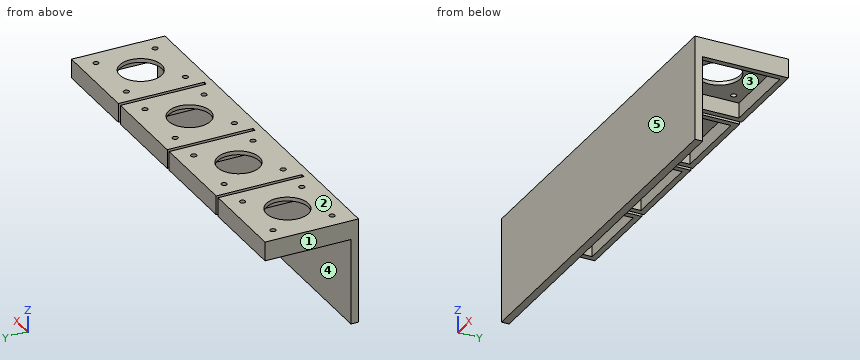
```python
from build123d import *

# Parameters (mm, degrees)
SKETCH_1_W           = 48
SKETCH_1_H           = 48
SKETCH_1_W_2         = 42
SKETCH_1_H_2         = 42
EXTRUDE_1_DEPTH      = 10
EXTRUDE_1_2_DEPTH    = 10
EXTRUDE_1_3_DEPTH    = 10
EXTRUDE_1_4_DEPTH    = 10
SKETCH_2_W           = 42
SKETCH_2_H           = 42
SKETCH_2_R           = 1.45
SKETCH_2_R_2         = 11
EXTRUDE_2_DEPTH      = 2
SKETCH_3_W           = 198
SKETCH_3_H           = 55
EXTRUDE_3_DEPTH      = 1
EXTRUDE_3_DEPTH_BACK = 3


with BuildPart() as part:
    # Sketch 1 → Extrude 1 (new body)
    with BuildSketch(Plane.XY):
        Rectangle(SKETCH_1_W, SKETCH_1_H)
        Rectangle(SKETCH_1_W_2, SKETCH_1_H_2, mode=Mode.SUBTRACT)
    extrude(amount=EXTRUDE_1_DEPTH)

    # Sketch 2 → Extrude 2 (add)
    with BuildSketch(Plane.XY.offset(10)):
        Rectangle(SKETCH_2_W, SKETCH_2_H)
        with Locations((-15.5, 15.5)):
            Circle(SKETCH_2_R, mode=Mode.SUBTRACT)
        with Locations((15.5, 15.5)):
            Circle(SKETCH_2_R, mode=Mode.SUBTRACT)
        with Locations((15.5, -15.5)):
            Circle(SKETCH_2_R, mode=Mode.SUBTRACT)
        with Locations((-15.5, -15.5)):
            Circle(SKETCH_2_R, mode=Mode.SUBTRACT)
        Circle(SKETCH_2_R_2, mode=Mode.SUBTRACT)
        with Locations((50, 0)):
            Rectangle(SKETCH_2_W, SKETCH_2_H)
        with Locations((34.5, 15.5)):
            Circle(SKETCH_2_R, mode=Mode.SUBTRACT)
        with Locations((65.5, 15.5)):
            Circle(SKETCH_2_R, mode=Mode.SUBTRACT)
        with Locations((65.5, -15.5)):
            Circle(SKETCH_2_R, mode=Mode.SUBTRACT)
        with Locations((34.5, -15.5)):
            Circle(SKETCH_2_R, mode=Mode.SUBTRACT)
        with Locations((50, 0)):
            Circle(SKETCH_2_R_2, mode=Mode.SUBTRACT)
        with Locations((100, 0)):
            Rectangle(SKETCH_2_W, SKETCH_2_H)
        with Locations((84.5, 15.5)):
            Circle(SKETCH_2_R, mode=Mode.SUBTRACT)
        with Locations((115.5, 15.5)):
            Circle(SKETCH_2_R, mode=Mode.SUBTRACT)
        with Locations((115.5, -15.5)):
            Circle(SKETCH_2_R, mode=Mode.SUBTRACT)
        with Locations((84.5, -15.5)):
            Circle(SKETCH_2_R, mode=Mode.SUBTRACT)
        with Locations((100, 0)):
            Circle(SKETCH_2_R_2, mode=Mode.SUBTRACT)
        with Locations((150, 0)):
            Rectangle(SKETCH_2_W, SKETCH_2_H)
        with Locations((134.5, 15.5)):
            Circle(SKETCH_2_R, mode=Mode.SUBTRACT)
        with Locations((165.5, 15.5)):
            Circle(SKETCH_2_R, mode=Mode.SUBTRACT)
        with Locations((165.5, -15.5)):
            Circle(SKETCH_2_R, mode=Mode.SUBTRACT)
        with Locations((134.5, -15.5)):
            Circle(SKETCH_2_R, mode=Mode.SUBTRACT)
        with Locations((150, 0)):
            Circle(SKETCH_2_R_2, mode=Mode.SUBTRACT)
    extrude(amount=-EXTRUDE_2_DEPTH)


with BuildPart() as body_2:
    # Sketch 1 → Extrude 1 2 (new body)
    with BuildSketch(Plane.XY):
        with Locations((50, 0)):
            Rectangle(SKETCH_1_W, SKETCH_1_H)
        with Locations((50, 0)):
            Rectangle(SKETCH_1_W_2, SKETCH_1_H_2, mode=Mode.SUBTRACT)
    extrude(amount=EXTRUDE_1_2_DEPTH)


with BuildPart() as body_3:
    # Sketch 1 → Extrude 1 3 (new body)
    with BuildSketch(Plane.XY):
        with Locations((100, 0)):
            Rectangle(SKETCH_1_W, SKETCH_1_H)
        with Locations((100, 0)):
            Rectangle(SKETCH_1_W_2, SKETCH_1_H_2, mode=Mode.SUBTRACT)
    extrude(amount=EXTRUDE_1_3_DEPTH)


with BuildPart() as body_4:
    # Sketch 1 → Extrude 1 4 (new body)
    with BuildSketch(Plane.XY):
        with Locations((150, 0)):
            Rectangle(SKETCH_1_W, SKETCH_1_H)
        with Locations((150, 0)):
            Rectangle(SKETCH_1_W_2, SKETCH_1_H_2, mode=Mode.SUBTRACT)
    extrude(amount=EXTRUDE_1_4_DEPTH)


with BuildPart() as extrude_2_piece_1:
    # of the separate pieces the step leaves, piece 1, a body of its own (extrude_2_pieces)
    add(part.part.solids().sort_by_distance((-24, -24, 0))[0])

    # Sketch 3 → Extrude 3 (add, two sides)
    with BuildSketch(Plane.XZ.offset(24)) as extrude_3_sk:
        with Locations((75, -17.5)):
            Rectangle(SKETCH_3_W, SKETCH_3_H)
    extrude(amount=EXTRUDE_3_DEPTH)
    extrude(extrude_3_sk.sketch, amount=-EXTRUDE_3_DEPTH_BACK)


with BuildPart() as extrude_2_piece_2:
    # of the separate pieces the step leaves, piece 2, a body of its own (extrude_2_pieces)
    add(part.part.solids().sort_by_distance((79, 21, 10))[0])


with BuildPart() as extrude_2_piece_3:
    # of the separate pieces the step leaves, piece 3, a body of its own (extrude_2_pieces)
    add(part.part.solids().sort_by_distance((29, 21, 10))[0])


with BuildPart() as extrude_2_piece_4:
    # of the separate pieces the step leaves, piece 4, a body of its own (extrude_2_pieces)
    add(part.part.solids().sort_by_distance((129, 21, 10))[0])


with BuildPart() as body_4_1:
    add(body_4.part)

    # Combine 1: union Extrude 2 piece 3, Extrude 2 piece 2, Extrude 2 piece 4, Extrude 2 piece 1, body 3, body 2
    add(extrude_2_piece_3.part)
    add(extrude_2_piece_2.part)
    add(extrude_2_piece_4.part)
    add(extrude_2_piece_1.part)
    add(body_3.part)
    add(body_2.part)


solid = body_4_1.part
```
Model file for the job. Use its own axes, mm. Face numbers are marked on the shaded views. A direction names the side the tool comes from. Give positions to 0.01 mm unless a question says otherwise; leave off trailing zeros. Order: outer loops, then holes, each group sorted by start corner. A loop starts at its lowest first (then second) coordinate and runs counter-clockwise, first axis right, second up.
1) 3-axis set-ups, long thin cutter, end or side, ignore diameter. For the marked faces 4 and 5: which of +Z, -Z, +X, -X, +Y, -Y reach the whole face in a straight line?
2) Saw through at B-B, the plane z = 5. Count the separate pieces of the cut face and the enclosed holes in it, then the cut area to 3 significant figures.
3) Saw through at C-C, the plane x = -7. Write the cut outline in (y, z), then the cut area to 3 significant figures.
4) Wall check: probe 1 along Y at (x, z) = (-15.5, 8.85); probe 2 along Y at (x, z) = (50, 8.95); probe 3 along Y at (x, z) = (70, 1). Give the ranges that are in metal, low to high.
5) Mould opens along X. For the marked faces 1, 2 and 3 say: +X half, -X half, draft (parallel to the pull), parting line (faces both ways), or undercut.
6) Pin check, flat tips, straight feed: pin 1 (13.5 mm diameter, centred on x = 100.5, y = -4, fed in from -Z) (3 decimals); pin 2 (1 mm diameter, centred on x = 70, y = 7.5, fed in from -Z). Stop position of each tip, or through.
7) Saw through at A-A, the plane x = 150. Write the cut outline in (y, z), then the cut area to 3 significant figures.
Computed:
1. face 4: -Z
1. face 5: +Z, -Z, +X, -X, -Y
2. separate pieces: 1
2. enclosed holes: 4
2. area: 2,380 mm2
3. outline: (-25, -45) - (-21, -45) - (-21, 8) - (-8.49, 8) - (-8.49, 10) - (-25, 10) - close; (8.49, 8) - (21, 8) - (21, 0) - (24, 0) - (24, 10) - (8.49, 10) - close
3. area: 300 mm2
4. probe 1: y = -25 to -16.95, -14.05 to 14.05, 16.95 to 24
4. probe 2: y = -25 to -11, 11 to 24
4. probe 3: y = -25 to -21, 21 to 24
5. face 1: -X half
5. face 2: draft
5. face 3: undercut
6. pin 1: passes through
6. pin 2: stops at z = 8
7. outline: (-25, -45) - (-21, -45) - (-21, 8) - (-11, 8) - (-11, 10) - (-25, 10) - close; (11, 8) - (21, 8) - (21, 0) - (24, 0) - (24, 10) - (11, 10) - close
7. area: 290 mm2
